Autodesk Inventor part; units mm, degrees
ref_plane "YZ Plane" through (0, 0, 0) normal (1, 0, 0) x (0, 1, 0)
ref_plane "XZ Plane" through (0, 0, 0) normal (0, 1, 0) x (-1, 0, 0)
ref_plane "XY Plane" through (0, 0, 0) normal (0, 0, 1) x (1, 0, 0)
sketch "Sketch1" plane through (0, 0, 0) normal (0, 0, 1) x (1, 0, 0)
  circle A0 centre (0, 0) radius 57.5
  dimension "d0" = 115
sketch "Sketch2" plane through (0, 0, 0) normal (1, 0, 0) x (0, 1, 0)
  line L0 (57.5, 0) -> (-57.5, 0) construction
  line L1 (-57.5, 0) -> (-57.5, 15)
  line L2 (-57.5, 15) -> (-39.5, 15)
  line L3 (-39.5, 15) -> (-39.5, 11)
  line L4 (-57.5, 0) -> (-52.5, 0)
  line L5 (-52.5, 0) -> (-52.5, 8)
  line L6 (-52.5, 8) -> (-50.42, 8)
  line L7 (-50.42, 8) -> (-50.42, 0)
  line L8 (-50.42, 0) -> (-45.42, 0)
  line L9 (-50.42, 0) -> (-45.42, 0) construction
  line L10 (-45.42, 0) -> (-45.42, 11)
  line L11 (-45.42, 11) -> (-39.5, 11)
  point P0 (0, 0)
  dimension "d1" = 15
  dimension "d3" = 4
  dimension "d4" = 90
  dimension "d5" = 5
  dimension "d6" = 8
  dimension "d7" = 2.08
  dimension "d8" = 5
  dimension "d9" = 0
  dimension "d10" = 90
  dimension "d15" = 13
sweep "Sweep1" add profiles "Sketch2" path "Sketch1"
sketch "Sketch3" plane through (0, 0, 15) normal (0, 0, 1) x (1, 0, 0)
  line L0 (56.5, 10) -> (-56.5, 10) construction
  line L1 (-56.5, 10) -> (-56.5, -10)
  line L2 (-56.5, -10) -> (56.5, -10) construction
  line L3 (56.5, -10) -> (56.5, 10)
  line L4 (56.5, 10) -> (-56.5, -10) construction
  arc A0 (-56.5, 10) -> (-56.5, -10) centre (-56.5, 0) ccw
  circle A1 centre (0, 0) radius 57.5 construction
  line L5 (-55.3308, 15.6447) -> (-55.3308, -15.6447)
  arc A2 (-55.3308, 15.6447) -> (-55.3308, -15.6447) centre (0, 0) ccw
  line L6 (0, 0) -> (-55.3308, -15.6447) construction
  line L7 (-55.3308, -15.6447) -> (-58.3308, -16.4929)
  line L8 (0, 0) -> (-55.3308, 15.6447) construction
  line L9 (-55.3308, 15.6447) -> (-58.3308, 16.4929)
  arc A3 (-58.3308, 16.4929) -> (-58.3308, -16.4929) centre (0, 0) ccw
  arc A4 (58.3308, -16.4929) -> (58.3308, 16.4929) centre (0, 0) ccw
  line L10 (55.3308, -15.6447) -> (58.3308, -16.4929)
  arc A5 (55.3308, -15.6447) -> (55.3308, 15.6447) centre (0, 0) ccw
  line L11 (55.3308, -15.6447) -> (55.3308, 15.6447)
  line L12 (55.3308, 15.6447) -> (58.3308, 16.4929)
  point P0 (-61.5, 0)
  dimension "d17" = 20
  dimension "d18" = 5
  dimension "d19" = 10
  dimension "d31" = 56.5
  dimension "d32" = 31.2894
  dimension "d33" = 3
  dimension "d34" = 3
  dimension "d37" = 360
extrude "Extrusion2" add sketch "Sketch3" against normal blind 4 contours L1 A0 A2 | A2 A0 A3 | A3 A0
hole "Hole1" at (-61.5, 0, 15) direction (0, 0, -1) diameter 3 end through all
extrude "Extrusion3" add sketch "Sketch3" along normal blind 4 and the other way blind 15 contours L10 A5 L12 A4 | L11 A5
extrude "Extrusion4" cut sketch "Sketch3" along normal blind 2.08 contours L11 A5
equation "\"d34\" = d33"
properties part number "Cap"
Check sheet for the modelled part. Datum: model origin and axes. Units: mm. A direction names the side the tool comes from. Round coordinates to 2 decimals unless told otherwise and drop trailing zeros. Order: outer loops, then holes, each group sorted by start corner. A loop starts at its lowest first (then second) coordinate and runs counter-clockwise, first axis right, second up. Notation, with made-up numbers: (32, 8) - (50, 8) arc R31 cw to (50, 37) - close; hole circle Ø3 at (-1.75, 43). An arc over 180 degrees is marked (long way). Write item = value, one per line.
Q1. Draft check along X on faces 1 (the face through (56.81, 16.063, 9.367)), 2 (the face through (-59, 0, 11)), 3 (the face through (60.617, 0.234, 9.367)), 4 (the face through (43.323, 13.643, 5.577)). Enter one of: pulls with the +X half, pulls with the -X half, needs draft (parallel to the pull), parting line crosses it, or undercut.
Computed:
face_1 = undercut
face_2 = needs draft
face_3 = pulls with the +X half
face_4 = undercut
Q2. Section check A-A (z = 3). State how many separate pieces and enclosed holes the cut face has, and give its area (3 significant figures).
Computed:
separate_pieces = 2
enclosed_holes = 2
area = 3,330 mm^2
Q3. Section check C-C (x = -61.5). Record the boundary of the cut face in (y, z), and give its area (3 significant figures).
Computed:
outline = (-8.66, 11) - (-1.5, 11) - (-1.5, 15) - (-8.66, 15) - close; (1.5, 11) - (8.66, 11) - (8.66, 15) - (1.5, 15) - close
area = 57.3 mm^2
Q4. Go/stop test with flat-tipped pins: pin 1 (11 mm diameter, centred on x = -61.5, y = -5, fed in from -Z); pin 2 (8 mm diameter, centred on x = -36.5, z = 17, fed in from +Y); pin 3 (10 mm diameter, centred on x = 16.5, z = 2.5, fed in from +Y); pin 4 (1 mm diameter, centred on y = -39.5, z = 16, fed in from -X). Record where each tip stops, or that it passes through.
Computed:
pin_1 = 0
pin_2 = 47.06
pin_3 = 56.34
pin_4 = through
Q5. Thickness scan on line 1 along Y through (x, z) = (0, 1.5); line 2 along Y through (x, z) = (0, 12.7); line 3 along X through (y, z) = (-25.5, 4.25). Record the ranges inside material, lowest first.
Computed:
line_1 = -57.5 to -52.5, -50.42 to -45.42, 45.42 to 50.42, 52.5 to 57.5
line_2 = -57.5 to -39.5, 39.5 to 57.5
line_3 = -51.54 to -45.89, -43.5 to -37.59, 37.59 to 43.5, 45.89 to 51.54
Q6. Tool access check on faces 5 (the face through (56.81, -16.063, 9.367)), 6 (the face through (-63, 0, 13)), 7 (the face through (50.076, 15.77, 4.056)). Record the directions out of +Z, -Z, +X, -X, +Y, -Y that give a thin tool (end or side, any length) a straight path to the whole face; none if there is none.
Computed:
face_5 = +Z, -Z, -Y
face_6 = +Z, -Z
face_7 = -Z
